Here's how the part is built. I have some questions about the finished solid (model axes, mm). A direction names the side the tool comes from. Coordinates: 2 decimals unless noted, no trailing zeros. Write each loop counter-clockwise with the first axis right and the second up, starting at its lowest first coordinate (ties: lowest second). Pieces come first, ordered by that corner, then holes. Notation, with made-up numbers: (-24, 45.5) -> (2, 45.5) arc R32 cw to (2, 80.5) -> close; hole circle Ø4 at (88, 6.5). An arc over 180 degrees is marked (long way). Use a Markdown table: item, result. Add a question column.
```python
from build123d import *

# Parameters (mm, degrees)
BOSS_EXTRUDE1_DEPTH = 5.08
FILLET1_R           = 2.54
SKETCH2_R           = 1.5625
CUT_EXTRUDE1_DEPTH  = 26.027057078


with BuildPart() as part:
    # Sketch1 → Boss-Extrude1 (new body)
    with BuildSketch(Plane.XY):
        with BuildLine():
            Line((18.669, -23.469960484), (12.319, -23.469960484))
            Line((12.319, -23.469960484), (12.319, -10.515960484))
            ThreePointArc((12.319, -10.515960484), (6.1595, -7.594960484), (0, -10.515960484))
            Line((0, -10.515960484), (0, -23.469960484))
            Line((0, -23.469960484), (-6.35, -23.469960484))
            Line((-6.35, -23.469960484), (-6.35, -22.199960484))
            Line((-6.35, -22.199960484), (-1.27, -22.199960484))
            Line((-1.27, -22.199960484), (-1.27, -10.515960484))
            ThreePointArc((-1.27, -10.515960484), (6.1595, -6.324960484), (13.589, -10.515960484))
            Line((13.589, -10.515960484), (13.589, -22.199960484))
            Line((13.589, -22.199960484), (18.669, -22.199960484))
            Line((18.669, -22.199960484), (18.669, -23.469960484))
        make_face()
    extrude(amount=BOSS_EXTRUDE1_DEPTH)

    # Fillet1
    fillet1_edges = [part.edges().sort_by_distance(p)[0] for p in [
        (-6.35, -22.834960484, 0),
        (-6.35, -22.834960484, 5.08),
        (18.669, -22.834960484, 0),
        (18.669, -22.834960484, 5.08),
    ]]
    fillet(fillet1_edges, radius=FILLET1_R - 0.0001)  # a hair under: the kernel refuses the full size

    # Sketch2 → Cut-Extrude1 (cut, through all)
    with BuildSketch(Plane(origin=(0, -22.199960484, 0), x_dir=(1, 0, 0), z_dir=(0, 1, 0))):
        with Locations(Location((16.129, -2.54, 0), (0, 0, 270))):
            Circle(SKETCH2_R)
        with Locations(Location((-3.81, -2.54, 0), (0, 0, 270))):
            Circle(SKETCH2_R)
    extrude(amount=-CUT_EXTRUDE1_DEPTH, mode=Mode.SUBTRACT)


solid = part.part
```
Q1. Suppose I cut it at D-D, the plane z = 4.65. Write out the boundary of the cut face in (x, y).
Q2. Please list where these lines run through material, in increasing order: line 1 (X direction, y = -23.05, z = 2.54); line 2 (X direction, y = -19.5, z = 2.65); line 3 (X direction, y = -22.25, z = 3.45).
Q3. Suppose I cut it at C-C, the plane z = 2.05. Write out the boundary of the cut face in (x, y).
Q4. Will these pins go through, and if not, where does the flat tip stop? pin 1 (1.5 mm diameter, centred on x = 12.5, z = 4, fed in from +Y); pin 2 (1.5 mm diameter, centred on y = -19, z = 3.5, fed in from -X); pin 3 (3 mm diameter, centred on x = 16, z = 4.5, fed in from +Y); pin 4 (3 mm diameter, centred on x = 16.129, z = 2.54, fed in from +Y).
Q5. Which directions (+Z, -Z, +X, -X, +Y, -Y) give clear straight access to the entire face, cutting with the end or side of a thin tool? Please do faces 4 (the flat face through (-2, -22.2, 3)), 5 (the flat face through (0, -17, 3)), 6 (the flat face through (15, -22.2, 4)), 7 (the cylindrical face through (-5.626, -22.826, 0.764)).
Q6. Suppose I cut it at A-A, the plane y = -16. Write out the boundary of the cut face in (x, z), and give its area (3 significant figures).
Q7. Suppose I cut it at B-B, the plane x = 15. Write out the boundary of the cut face in (y, z), and give its area (3 significant figures).
Q8. Thinking about a two-plate mould opening in X: for faces 1 (the cylindrical face through (17.94, -22.84, 4.32)), 2 (the cylindrical face through (6.258, -7.596, 2.504)), 3 (the flat face through (-1.27, -16, 3)), which applies, released by +X, released by -X, zero draft, split by the parting line, or undercut?
Answer key:
| question | item | result |
|---|---|---|
| 1 | outline | (-5.22, -23.47) -> (0, -23.47) -> (0, -10.52) arc R7.95 cw to (12.32, -10.52) -> (12.32, -23.47) -> (17.54, -23.47) -> (17.54, -22.2) -> (13.59, -22.2) -> (13.59, -10.52) arc R8.68 ccw to (-1.27, -10.52) -> (-1.27, -22.2) -> (-5.22, -22.2) -> close |
| 2 | line 1 | x = -6.35 to -5.37, -2.25 to 0, 12.32 to 14.57, 17.69 to 18.67 |
| 2 | line 2 | x = -1.27 to 0, 12.32 to 13.59 |
| 2 | line 3 | x = -6.18 to -5.08, -2.54 to 0, 12.32 to 14.86, 17.4 to 18.5 |
| 3 | outline | (-6.3, -23.47) -> (-5.29, -23.47) -> (-5.29, -22.2) -> (-6.3, -22.2) -> close; (-2.33, -23.47) -> (0, -23.47) -> (0, -10.52) arc R7.95 cw to (12.32, -10.52) -> (12.32, -23.47) -> (14.65, -23.47) -> (14.65, -22.2) -> (13.59, -22.2) -> (13.59, -10.52) arc R8.68 ccw to (-1.27, -10.52) -> (-1.27, -22.2) -> (-2.33, -22.2) -> close; (17.61, -23.47) -> (18.62, -23.47) -> (18.62, -22.2) -> (17.61, -22.2) -> close |
| 4 | pin 1 | stops at y = -8.36 |
| 4 | pin 2 | stops at x = -1.27 |
| 4 | pin 3 | stops at y = -22.2 |
| 4 | pin 4 | passes through |
| 5 | face 4 | +Z, -Z, -X, +Y |
| 5 | face 5 | +Z, -Z, -Y |
| 5 | face 6 | +Z, -Z, +X, +Y |
| 5 | face 7 | -Z, -X, +Y, -Y |
| 6 | outline | (-1.27, 0) -> (0, 0) -> (0, 5.08) -> (-1.27, 5.08) -> close; (12.32, 0) -> (13.59, 0) -> (13.59, 5.08) -> (12.32, 5.08) -> close |
| 6 | area | 12.9 mm^2 |
| 7 | outline | (-23.47, 0) -> (-22.2, 0) -> (-22.2, 1.46) -> (-23.47, 1.46) -> close; (-23.47, 3.62) -> (-22.2, 3.62) -> (-22.2, 5.08) -> (-23.47, 5.08) -> close |
| 7 | area | 3.71 mm^2 |
| 8 | face 1 | released by +X |
| 8 | face 2 | undercut |
| 8 | face 3 | released by -X |
